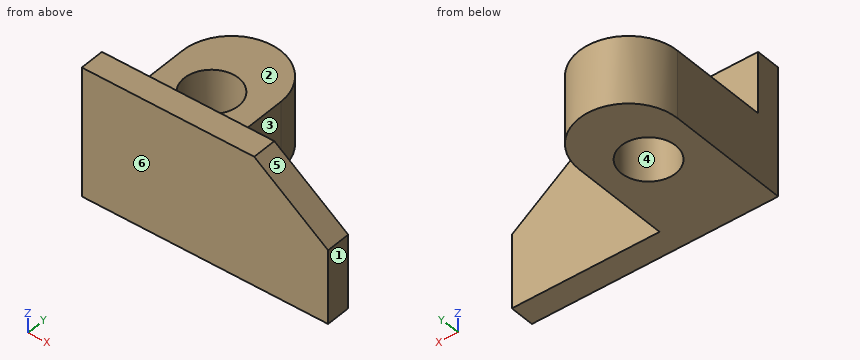
from build123d import *

# Parameters (mm, degrees)
BOSS_EXTRUDE1_DEPTH = 20
SKETCH4_W           = 80
SKETCH4_H           = 55
BOSS_EXTRUDE3_DEPTH = 120
FILLET2_RADIUS      = 40
FILLET2_LENGTH      = 55
SKETCH5_R           = 22
CUT_EXTRUDE1_DEPTH  = 120


with BuildPart() as part:
    # Sketch1 → Boss-Extrude1 (new body)
    with BuildSketch(Plane(origin=(0, 0, 0), x_dir=(1, 0, 0), z_dir=(0, 1, 0))):
        Polygon((-200, 60), (0, 60), (0, 0), (-60, -45), (-200, -45), align=None)
    extrude(amount=BOSS_EXTRUDE1_DEPTH)

    # Sketch4 → Boss-Extrude3 (add)
    with BuildSketch(Plane(origin=(0, 20, 0), x_dir=(1, 0, 0), z_dir=(0, 1, 0))):
        with Locations((-160, 32.5)):
            Rectangle(SKETCH4_W, SKETCH4_H)
    extrude(amount=BOSS_EXTRUDE3_DEPTH)

    # Fillet2: full round fillet: the end face becomes a half cylinder, R = half its width
    fillet2_face = Plane((-160, 140, -32.5), x_dir=(0, 0, 1), z_dir=(0, 1, 0))  # on the end face: x along it, z out of the body
    fillet2_slab = fillet2_face.offset(-FILLET2_RADIUS / 2) * Box(FILLET2_LENGTH, 2 * FILLET2_RADIUS, FILLET2_RADIUS, mode=Mode.PRIVATE)  # the body's end, R deep
    fillet2_round = Plane((-160, 100, -32.5), x_dir=(0, 1, 0), z_dir=(0, 0, 1)) * Cylinder(FILLET2_RADIUS, FILLET2_LENGTH, mode=Mode.PRIVATE)  # its axis R under the face
    add(fillet2_slab - fillet2_round, mode=Mode.SUBTRACT)

    # Sketch5 → Cut-Extrude1 (cut)
    with BuildSketch(Plane.XY.offset(-5)):
        with Locations((-160, 80)):
            Circle(SKETCH5_R)
    extrude(amount=-CUT_EXTRUDE1_DEPTH, mode=Mode.SUBTRACT)


solid = part.part
The listing builds one solid part. Answer for the finished solid, in the listing's coordinates (mm). Face numbers are marked on the shaded views. A direction names the side the tool comes from. Give positions to 0.01 mm unless a question says otherwise; leave off trailing zeros. Write each loop counter-clockwise with the first axis right and the second up, starting at its lowest first coordinate (ties: lowest second). Pieces come first, ordered by that corner, then holes.
1) Given P1, Ø10, axis at x = -112, y = 31, coming from the -Z side; P2, Ø2, axis at x = -137, y = 83.5, coming from the +Z side; P3, Ø6, axis at x = -132.5, z = -32, coming from the +Y side; P4, Ø2, axis at x = -54.5, z = -43, coming from the +Y side, each flat-ended and moving along its own axis, determine where each tip first touches the part or whether it passes through.
2) Find the intervals of material crossed by L1, parallel to Y at x = -160, z = -21; L2, parallel to Y at x = -102.5, z = -12.5; L3, parallel to Z at x = -126.5, y = 82, in increasing order.
3) Section C-C (z = -22) is taken. Write down the section's boundary in (x, y).
4) Section B-B (y = 80) is taken. Write down the section's boundary in (x, z), and give its area (3 significant figures).
5) Section D-D (x = -53) is taken. Write down the section's boundary in (y, z).
6) A tool of negligible diameter and unlimited length cuts with its end or side. For the marked faces 1, 2 and 3, from which of +Z, -Z, +X, -X, +Y, -Y can it reach the whole face along a straight path? Write none if from no direction.
7) Section A-A (x = -160) is taken. Write down the section's boundary in (y, z), and give its area (3 significant figures).
8) For a pull along Y with two mould halves and no side action, classify the marked faces 4, 5 and 6 as pulls with the +Y half, pulls with the -Y half, needs draft (parallel to the pull), parting line crosses it, or undercut.
Response:
1. P1: passes through
1. P2: stops at z = -5
1. P3: stops at y = 131.62
1. P4: stops at y = 20
2. L1: y = 0 to 58, 102 to 140
2. L2: y = 0 to 20
2. L3: z = -60 to -5
3. outline: (-200, 0) - (0, 0) - (0, 20) - (-120, 20) - (-120, 100) arc R40 ccw to (-200, 100) - close; hole circle Ø44 at (-160, 80)
4. outline: (-200, -60) - (-182, -60) - (-182, -5) - (-200, -5) - close; (-138, -60) - (-120, -60) - (-120, -5) - (-138, -5) - close
4. area: 1,980 mm2
5. outline: (0, -60) - (20, -60) - (20, 39.75) - (0, 39.75) - close
6. face 1: +Z, -Z, +X, +Y, -Y
6. face 2: +Z, +X, -X, +Y
6. face 3: +Z, -Z, +X, +Y
7. outline: (0, -60) - (58, -60) - (58, -5) - (20, -5) - (20, 45) - (0, 45) - close; (102, -60) - (140, -60) - (140, -5) - (102, -5) - close
7. area: 6,280 mm2
8. face 4: undercut
8. face 5: needs draft
8. face 6: pulls with the -Y half
